The listing builds one solid part. Answer for the finished solid, in the listing's coordinates (mm). Face numbers are marked on the shaded views. A direction names the side the tool comes from. Round coordinates to 2 decimals unless told otherwise and drop trailing zeros. Write each loop counter-clockwise with the first axis right and the second up, starting at its lowest first coordinate (ties: lowest second). Pieces come first, ordered by that corner, then holes. Notation, with made-up numbers: M 10,-9 L 27,-9 A21 cw 27,14 Z; hole C 82,-21 d9. An arc over 180 degrees is marked long. One line per item, written item: value. Start each with the question number.
(1) Consider probe 1 along Y at (x, z) = (0, 1.25); probe 2 along X at (y, z) = (-24, 2.75); probe 3 along X at (y, z) = (5.5, 1.75). Determine where each line is inside the solid, lowest interval first.
(2) For the marked faces 3 and 4, determine the directions among +Z, -Z, +X, -X, +Y, -Y from which every point of the face is accessible in a straight line to the end or side of a thin tool.
(3) For a pull along X with two mould halves and no side action, classify the marked faces 1 and 2 as released by +X, released by -X, zero draft, split by the parting line, or undercut.
(4) Section B-B (y = 0) is taken. Determine the outline of the cut face in (x, z).
(5) Section A-A (x = 0) is taken. Determine the outline of the cut face in (y, z), plus the area to 3 significant figures.
(6) Given P1, Ø3.5, axis at x = 0, y = 0, coming from the -Z side; P2, Ø4, axis at x = 10.5, z = 2.5, coming from the +Y side, each flat-ended and moving along its own axis, determine where each tip first touches the part or whether it passes through.
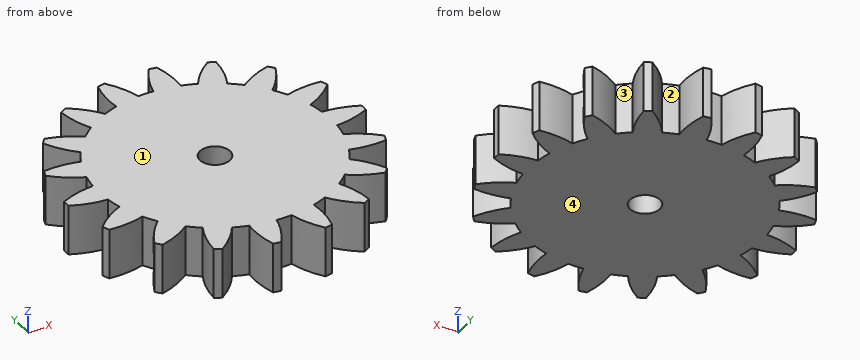
```python
from build123d import *

# Parameters (mm, degrees)
SKETCH1_R           = 3
BOSS_EXTRUDE1_DEPTH = 10


with BuildPart() as part:
    # Sketch1 → Boss-Extrude1 (new body)
    with BuildSketch(Plane.XY):
        with BuildLine():
            ThreePointArc((-6.504789318, 22.320477525), (-7.951626312, 21.846913741), (-9.364368684, 21.279675753))
            add(Edge.make_bspline(
                [(-14.34407304, 26.348578114), (-11.348209695, 24.318322412), (-9.364368684, 21.279675753)],
                knots=[0, 0, 0, 1, 1, 1], degree=2))
            ThreePointArc((-14.34407304, 26.348578114), (-15, 25.980762114), (-15.646501481, 25.596620703))
            add(Edge.make_bspline(
                [(-15.646501481, 25.596620703), (-15.386180139, 21.98699909), (-13.746555444, 18.749619047)],
                knots=[0, 0, 0, 1, 1, 1], degree=2))
            ThreePointArc((-13.746555444, 18.749619047), (-14.944169138, 17.809767258), (-16.077705902, 16.793551558))
            add(Edge.make_bspline(
                [(-22.49076405, 19.853602505), (-18.981185027, 18.970431814), (-16.077705902, 16.793551558)],
                knots=[0, 0, 0, 1, 1, 1], degree=2))
            ThreePointArc((-22.49076405, 19.853602505), (-22.981333294, 19.283628291), (-23.457461864, 18.701536913))
            add(Edge.make_bspline(
                [(-23.457461864, 18.701536913), (-21.978276518, 15.398637262), (-19.330284106, 12.917279798)],
                knots=[0, 0, 0, 1, 1, 1], degree=2))
            ThreePointArc((-19.330284106, 12.917279798), (-20.134224613, 11.6245), (-20.851834506, 10.281877199))
            add(Edge.make_bspline(
                [(-27.924736988, 10.963989426), (-24.324749311, 11.334427165), (-20.851834506, 10.281877199)],
                knots=[0, 0, 0, 1, 1, 1], degree=2))
            ThreePointArc((-27.924736988, 10.963989426), (-28.190778624, 10.2606043), (-28.439106151, 9.550771765))
            add(Edge.make_bspline(
                [(-28.439106151, 9.550771765), (-25.919468385, 6.95297252), (-22.58249522, 5.526925967)],
                knots=[0, 0, 0, 1, 1, 1], degree=2))
            ThreePointArc((-22.58249522, 5.526925967), (-22.89579545, 4.037146483), (-23.110924128, 2.530056705))
            add(Edge.make_bspline(
                [(-29.99057452, 0.751957411), (-26.734389834, 2.331323322), (-23.110924128, 2.530056705)],
                knots=[0, 0, 0, 1, 1, 1], degree=2))
            ThreePointArc((-29.99057452, 0.751957411), (-30, 0), (-29.99057452, -0.751957411))
            add(Edge.make_bspline(
                [(-29.99057452, -0.751957411), (-26.734389834, -2.331323322), (-23.110924128, -2.530056705)],
                knots=[0, 0, 0, 1, 1, 1], degree=2))
            ThreePointArc((-23.110924128, -2.530056705), (-22.89579545, -4.037146483), (-22.58249522, -5.526925967))
            add(Edge.make_bspline(
                [(-28.439106151, -9.550771765), (-25.919468385, -6.95297252), (-22.58249522, -5.526925967)],
                knots=[0, 0, 0, 1, 1, 1], degree=2))
            ThreePointArc((-28.439106151, -9.550771765), (-28.190778624, -10.2606043), (-27.924736988, -10.963989426))
            add(Edge.make_bspline(
                [(-27.924736988, -10.963989426), (-24.324749311, -11.334427165), (-20.851834506, -10.281877199)],
                knots=[0, 0, 0, 1, 1, 1], degree=2))
            ThreePointArc((-20.851834506, -10.281877199), (-20.134224613, -11.6245), (-19.330284106, -12.917279798))
            add(Edge.make_bspline(
                [(-23.457461864, -18.701536913), (-21.978276518, -15.398637262), (-19.330284106, -12.917279798)],
                knots=[0, 0, 0, 1, 1, 1], degree=2))
            ThreePointArc((-23.457461864, -18.701536913), (-22.981333294, -19.283628291), (-22.49076405, -19.853602505))
            add(Edge.make_bspline(
                [(-22.49076405, -19.853602505), (-18.981185027, -18.970431814), (-16.077705902, -16.793551558)],
                knots=[0, 0, 0, 1, 1, 1], degree=2))
            ThreePointArc((-16.077705902, -16.793551558), (-14.944169138, -17.809767258), (-13.746555444, -18.749619047))
            add(Edge.make_bspline(
                [(-15.646501481, -25.596620703), (-15.386180139, -21.98699909), (-13.746555444, -18.749619047)],
                knots=[0, 0, 0, 1, 1, 1], degree=2))
            ThreePointArc((-15.646501481, -25.596620703), (-15, -25.980762114), (-14.34407304, -26.348578114))
            add(Edge.make_bspline(
                [(-14.34407304, -26.348578114), (-11.348209695, -24.318322412), (-9.364368684, -21.279675753)],
                knots=[0, 0, 0, 1, 1, 1], degree=2))
            ThreePointArc((-9.364368684, -21.279675753), (-7.951626312, -21.846913741), (-6.504789318, -22.320477525))
            add(Edge.make_bspline(
                [(-5.948342101, -29.404374271), (-6.938283358, -25.923404334), (-6.504789318, -22.320477525)],
                knots=[0, 0, 0, 1, 1, 1], degree=2))
            ThreePointArc((-5.948342101, -29.404374271), (-5.20944533, -29.54423259), (-4.467275124, -29.665526339))
            add(Edge.make_bspline(
                [(-4.467275124, -29.665526339), (-2.346472793, -26.733064427), (-1.5215504, -23.199156997)],
                knots=[0, 0, 0, 1, 1, 1], degree=2))
            ThreePointArc((-1.5215504, -23.199156997), (0, -23.249), (1.5215504, -23.199156997))
            add(Edge.make_bspline(
                [(4.467275124, -29.665526339), (2.346472793, -26.733064427), (1.5215504, -23.199156997)],
                knots=[0, 0, 0, 1, 1, 1], degree=2))
            ThreePointArc((4.467275124, -29.665526339), (5.20944533, -29.54423259), (5.948342101, -29.404374271))
            add(Edge.make_bspline(
                [(5.948342101, -29.404374271), (6.938283358, -25.923404334), (6.504789318, -22.320477525)],
                knots=[0, 0, 0, 1, 1, 1], degree=2))
            ThreePointArc((6.504789318, -22.320477525), (7.951626312, -21.846913741), (9.364368684, -21.279675753))
            add(Edge.make_bspline(
                [(14.34407304, -26.348578114), (11.348209695, -24.318322412), (9.364368684, -21.279675753)],
                knots=[0, 0, 0, 1, 1, 1], degree=2))
            ThreePointArc((14.34407304, -26.348578114), (15, -25.980762114), (15.646501481, -25.596620703))
            add(Edge.make_bspline(
                [(15.646501481, -25.596620703), (15.386180139, -21.98699909), (13.746555444, -18.749619047)],
                knots=[0, 0, 0, 1, 1, 1], degree=2))
            ThreePointArc((13.746555444, -18.749619047), (14.944169138, -17.809767258), (16.077705902, -16.793551558))
            add(Edge.make_bspline(
                [(22.49076405, -19.853602505), (18.981185027, -18.970431814), (16.077705902, -16.793551558)],
                knots=[0, 0, 0, 1, 1, 1], degree=2))
            ThreePointArc((22.49076405, -19.853602505), (22.981333294, -19.283628291), (23.457461864, -18.701536913))
            add(Edge.make_bspline(
                [(23.457461864, -18.701536913), (21.978276518, -15.398637262), (19.330284106, -12.917279798)],
                knots=[0, 0, 0, 1, 1, 1], degree=2))
            ThreePointArc((19.330284106, -12.917279798), (20.134224613, -11.6245), (20.851834506, -10.281877199))
            add(Edge.make_bspline(
                [(27.924736988, -10.963989426), (24.324749311, -11.334427165), (20.851834506, -10.281877199)],
                knots=[0, 0, 0, 1, 1, 1], degree=2))
            ThreePointArc((27.924736988, -10.963989426), (28.190778624, -10.2606043), (28.439106151, -9.550771765))
            add(Edge.make_bspline(
                [(28.439106151, -9.550771765), (25.919468385, -6.95297252), (22.58249522, -5.526925967)],
                knots=[0, 0, 0, 1, 1, 1], degree=2))
            ThreePointArc((22.58249522, -5.526925967), (22.89579545, -4.037146483), (23.110924128, -2.530056705))
            add(Edge.make_bspline(
                [(29.99057452, -0.751957411), (26.734389834, -2.331323322), (23.110924128, -2.530056705)],
                knots=[0, 0, 0, 1, 1, 1], degree=2))
            ThreePointArc((29.99057452, -0.751957411), (30, 0), (29.99057452, 0.751957411))
            add(Edge.make_bspline(
                [(29.99057452, 0.751957411), (26.734389834, 2.331323322), (23.110924128, 2.530056705)],
                knots=[0, 0, 0, 1, 1, 1], degree=2))
            ThreePointArc((23.110924128, 2.530056705), (22.89579545, 4.037146483), (22.58249522, 5.526925967))
            add(Edge.make_bspline(
                [(28.439106151, 9.550771765), (25.919468385, 6.95297252), (22.58249522, 5.526925967)],
                knots=[0, 0, 0, 1, 1, 1], degree=2))
            ThreePointArc((28.439106151, 9.550771765), (28.190778624, 10.2606043), (27.924736988, 10.963989426))
            add(Edge.make_bspline(
                [(27.924736988, 10.963989426), (24.324749311, 11.334427165), (20.851834506, 10.281877199)],
                knots=[0, 0, 0, 1, 1, 1], degree=2))
            ThreePointArc((20.851834506, 10.281877199), (20.134224613, 11.6245), (19.330284106, 12.917279798))
            add(Edge.make_bspline(
                [(23.457461864, 18.701536913), (21.978276518, 15.398637262), (19.330284106, 12.917279798)],
                knots=[0, 0, 0, 1, 1, 1], degree=2))
            ThreePointArc((23.457461864, 18.701536913), (22.981333294, 19.283628291), (22.49076405, 19.853602505))
            add(Edge.make_bspline(
                [(22.49076405, 19.853602505), (18.981185027, 18.970431814), (16.077705902, 16.793551558)],
                knots=[0, 0, 0, 1, 1, 1], degree=2))
            ThreePointArc((16.077705902, 16.793551558), (14.944169138, 17.809767258), (13.746555444, 18.749619047))
            add(Edge.make_bspline(
                [(15.646501481, 25.596620703), (15.386180139, 21.98699909), (13.746555444, 18.749619047)],
                knots=[0, 0, 0, 1, 1, 1], degree=2))
            ThreePointArc((15.646501481, 25.596620703), (15, 25.980762114), (14.34407304, 26.348578114))
            add(Edge.make_bspline(
                [(14.34407304, 26.348578114), (11.348209695, 24.318322412), (9.364368684, 21.279675753)],
                knots=[0, 0, 0, 1, 1, 1], degree=2))
            ThreePointArc((9.364368684, 21.279675753), (7.951626312, 21.846913741), (6.504789318, 22.320477525))
            add(Edge.make_bspline(
                [(5.948342101, 29.404374271), (6.938283358, 25.923404334), (6.504789318, 22.320477525)],
                knots=[0, 0, 0, 1, 1, 1], degree=2))
            ThreePointArc((5.948342101, 29.404374271), (5.20944533, 29.54423259), (4.467275124, 29.665526339))
            add(Edge.make_bspline(
                [(4.467275124, 29.665526339), (2.346472793, 26.733064427), (1.5215504, 23.199156997)],
                knots=[0, 0, 0, 1, 1, 1], degree=2))
            ThreePointArc((1.5215504, 23.199156997), (0, 23.249), (-1.5215504, 23.199156997))
            add(Edge.make_bspline(
                [(-4.467275124, 29.665526339), (-2.346472793, 26.733064427), (-1.5215504, 23.199156997)],
                knots=[0, 0, 0, 1, 1, 1], degree=2))
            ThreePointArc((-4.467275124, 29.665526339), (-5.20944533, 29.54423259), (-5.948342101, 29.404374271))
            add(Edge.make_bspline(
                [(-5.948342101, 29.404374271), (-6.938283358, 25.923404334), (-6.504789318, 22.320477525)],
                knots=[0, 0, 0, 1, 1, 1], degree=2))
        make_face()
        Circle(SKETCH1_R, mode=Mode.SUBTRACT)
    extrude(amount=BOSS_EXTRUDE1_DEPTH)


solid = part.part
```
Recorded:
1. probe 1: y = -23.25 to -3, 3 to 23.25
1. probe 2: x = -15.46 to -11.54, -6.63 to -1.73, 1.73 to 6.63, 11.54 to 15.46
1. probe 3: x = -22.59 to 22.59
2. face 3: +Z, -Z
2. face 4: -Z, +X, -X, +Y, -Y
3. face 1: zero draft
3. face 2: undercut
4. outline: M -30,0 L -3,0 L -3,10 L -30,10 Z; M 3,0 L 30,0 L 30,10 L 3,10 Z
5. outline: M -23.25,0 L -3,0 L -3,10 L -23.25,10 Z; M 3,0 L 23.25,0 L 23.25,10 L 3,10 Z
5. area: 405 mm2
6. P1: passes through
6. P2: stops at y = 24.92
